The listing builds one solid part. Answer for the finished solid, in the listing's coordinates (mm). Give positions to 0.01 mm unless a question says otherwise; leave off trailing zeros. Loops run counter-clockwise (first coordinate to the right, second up) from the corner with the lowest first, then second, coordinate; pieces in that order, holes last.
Item 1: Section B-B, the plane y = 1.27 is taken. Give the vertices of the cut face in (x, z) (3 decimals), and give its area (3 significant figures).
Item 2: The mould has two halves that part along Y. Classify faces 1 (the face through (-3.81, 0, 0)), 2 (the face through (0, -5.08, 0)), 3 (the face through (0, 5.08, 0)): pulls with the +Y half, pulls with the -Y half, needs draft (parallel to the pull), parting line crosses it, or undercut.
Item 3: Section C-C, the plane y = -2 is taken. Give the vertices of the cut face in (x, z) (3 decimals), and give its area (3 significant figures).
Item 4: Section A-A, the plane x = 0 is taken. Give the vertices of the cut face in (y, z) (3 decimals).
Item 5: Consider line 1 along Z through (x, y) = (3, 1.25) (3 decimals); line 2 along Z through (x, y) = (-0.75, 4) (3 decimals); line 3 along X through (y, z) = (-4, 3.5). Determine where each line is inside the solid, lowest interval first.
Item 6: Section D-D, the plane x = -1.5 is taken. Give the vertices of the cut face in (y, z) (3 decimals).
Item 7: This flat-tipped pin is pushed along its axis until it touches: pin 1 Ø4 at (x, y) = (0.5, 1) entering from +Z. Where does it stop, or does it pass through?
Autodesk Inventor part; units mm, degrees
ref_plane "YZ Plane" through (0, 0, 0) normal (1, 0, 0) x (0, 1, 0)
ref_plane "XZ Plane" through (0, 0, 0) normal (0, 1, 0) x (-1, 0, 0)
ref_plane "XY Plane" through (0, 0, 0) normal (0, 0, 1) x (1, 0, 0)
sketch "Sketch1" plane through (0, 0, 0) normal (0, 0, 1) x (1, 0, 0)
  line L0 (-3.81, 5.08) -> (3.81, 5.08)
  line L1 (3.81, 5.08) -> (3.81, -5.08)
  line L2 (3.81, -5.08) -> (-3.81, -5.08)
  line L3 (-3.81, -5.08) -> (-3.81, 5.08)
  line L4 (0, 0) -> (0, 5.08) construction
  line L5 (0, 0) -> (0, -5.08) construction
  line L6 (0, 0) -> (-3.81, 0) construction
  line L7 (0, 0) -> (3.81, 0) construction
  dimension "d0" = 7.62
  dimension "d1" = 10.16
extrude "Extrusion1" add sketch "Sketch1" along normal mid plane 6.35
sketch "Sketch2" plane through (0, 0, 3.175) normal (0, 0, 1) x (1, 0, 0)
  line L0 (-3.81, 5.08) -> (3.81, 5.08)
  line L1 (3.81, -5.08) -> (-3.81, -5.08)
  line L2 (0, 5.08) -> (0, -5.08) construction
  circle A0 centre (0, 3.81) radius 0.889
  line L3 (-3.81, -5.08) -> (-3.81, 5.08)
  circle A1 centre (0, 1.27) radius 0.889
  circle A2 centre (0, -1.27) radius 0.889
  circle A3 centre (0, -3.81) radius 0.889
  dimension "d4" = 1.27
  dimension "d5" = 1.778
  dimension "d14" = 2.54
extrude "Extrusion2" add sketch "Sketch2" along normal blind 1.016 contours A0
fillet "Fillet1" radius 0.889 1 edges at (-0.889, 3.81, 4.191)
extrude "Extrusion3" add sketch "Sketch2" along normal blind 1.016 contours A1
fillet "Fillet2" radius 0.889 1 edges at (-0.889, 1.27, 4.191)
extrude "Extrusion4" add sketch "Sketch2" along normal blind 1.016 contours A2
fillet "Fillet3" radius 0.889 1 edges at (-0.889, -1.27, 4.191)
extrude "Extrusion5" add sketch "Sketch2" along normal blind 1.016 contours A3
fillet "Fillet4" radius 0.889 1 edges at (-0.889, -3.81, 4.191)
properties part number "cRIO-FRC LED"
Worked answers:
1. outline: (-3.81, -3.175) - (3.81, -3.175) - (3.81, 3.175) - (0.889, 3.175) - (0.889, 3.302) arc R0.889 ccw to (-0.889, 3.302) - (-0.889, 3.175) - (-3.81, 3.175) - close
1. area: 49.9 mm2
2. face 1: needs draft
2. face 2: pulls with the -Y half
2. face 3: pulls with the +Y half
3. outline: (-3.81, -3.175) - (3.81, -3.175) - (3.81, 3.175) - (0.507, 3.175) - (0.507, 3.302) arc R0.507 ccw to (-0.507, 3.302) - (-0.507, 3.175) - (-3.81, 3.175) - close
3. area: 48.9 mm2
4. outline: (-5.08, -3.175) - (5.08, -3.175) - (5.08, 3.175) - (4.699, 3.175) - (4.699, 3.302) arc R0.889 ccw to (2.921, 3.302) - (2.921, 3.175) - (2.159, 3.175) - (2.159, 3.302) arc R0.889 ccw to (0.381, 3.302) - (0.381, 3.175) - (-0.381, 3.175) - (-0.381, 3.302) arc R0.889 ccw to (-2.159, 3.302) - (-2.159, 3.175) - (-2.921, 3.175) - (-2.921, 3.302) arc R0.889 ccw to (-4.699, 3.302) - (-4.699, 3.175) - (-5.08, 3.175) - close
5. line 1: z = -3.175 to 3.175
5. line 2: z = -3.175 to 3.74
5. line 3: x = -0.85 to 0.85
6. outline: (-5.08, -3.175) - (5.08, -3.175) - (5.08, 3.175) - (-5.08, 3.175) - close
7. pin 1: stops at z = 4.19
